Build history of the part. All positions in model axes, mm. A direction names the side the tool comes from. Round coordinates to 2 decimals unless told otherwise and drop trailing zeros. Order: outer loops, then holes, each group sorted by start corner. A loop starts at its lowest first (then second) coordinate and runs counter-clockwise, first axis right, second up. Notation, with made-up numbers: (22.25, 2.25) -> (59.25, 2.25) arc R30 ccw to (59.25, 33.25) -> close; hole circle Ø8 at (75, 81.25). An arc over 180 degrees is marked (long way). Answer as a JSON object with one key per item and string values.
from build123d import *

# Parameters (mm, degrees)
F0_W      = 85
F0_H      = 85
F0_R      = 2
F3_DEPTH  = 18.5
F4_DEPTH  = 14
F5_R      = 5
F6_R      = 3
F7_R      = 1
F8_R      = 3.1
F9_DEPTH  = 3.1
F10_R     = 3.1
F11_DEPTH = 3.1
F12_R     = 3.1
F13_DEPTH = 3.1
F14_R     = 3.1
F15_DEPTH = 3.1
F16_DEPTH = 1
F17_ANGLE = 180


# Not quite as in the source:
# - a feature names something its author has since deleted; it is built from what else it names


with BuildPart() as f3:
    # F0 (on Top) → F3 (new body)
    with BuildSketch(Plane.XY):
        Rectangle(F0_W, F0_H)
        with Locations((0, -37.75)):
            Circle(F0_R, mode=Mode.SUBTRACT)
        with BuildLine():
            ThreePointArc((-33, 30), (-32.1213203436, 32.1213203436), (-30, 33))
            Line((-30, 33), (30, 33))
            ThreePointArc((30, 33), (32.1213203436, 32.1213203436), (33, 30))
            Line((33, 30), (33, -30))
            ThreePointArc((33, -30), (32.1213203436, -32.1213203436), (30, -33))
            Line((30, -33), (-30, -33))
            ThreePointArc((-30, -33), (-32.1213203436, -32.1213203436), (-33, -30))
            Line((-33, -30), (-33, 30))
        make_face(mode=Mode.SUBTRACT)
        with BuildLine():
            Line((30, 33), (-30, 33))
            ThreePointArc((-30, 33), (-32.1213203436, 32.1213203436), (-33, 30))
            Line((-33, 30), (-33, -30))
            ThreePointArc((-33, -30), (-32.1213203436, -32.1213203436), (-30, -33))
            Line((-30, -33), (30, -33))
            ThreePointArc((30, -33), (32.1213203436, -32.1213203436), (33, -30))
            Line((33, -30), (33, 30))
            ThreePointArc((33, 30), (32.1213203436, 32.1213203436), (30, 33))
        make_face()
        with Locations((0, -37.75)):
            Circle(F0_R)
    extrude(amount=F3_DEPTH)

    # F0 (on Top) → F4 (cut)
    with BuildSketch(Plane.XY):
        with BuildLine():
            Line((30, 33), (-30, 33))
            ThreePointArc((-30, 33), (-32.1213203436, 32.1213203436), (-33, 30))
            Line((-33, 30), (-33, -30))
            ThreePointArc((-33, -30), (-32.1213203436, -32.1213203436), (-30, -33))
            Line((-30, -33), (30, -33))
            ThreePointArc((30, -33), (32.1213203436, -32.1213203436), (33, -30))
            Line((33, -30), (33, 30))
            ThreePointArc((33, 30), (32.1213203436, 32.1213203436), (30, 33))
        make_face()
    extrude(amount=F4_DEPTH, mode=Mode.SUBTRACT)

    # F5
    f5_edges = [f3.edges().sort_by_distance(p)[0] for p in [
        (0, 42.5, 18.5),
        (-42.5, 0, 18.5),
        (0, -42.5, 18.5),
        (42.5, 0, 18.5),
        (42.5, 42.5, 9.25),
        (-42.5, 42.5, 9.25),
        (-42.5, -42.5, 9.25),
        (42.5, -42.5, 9.25),
    ]]
    fillet(f5_edges, radius=F5_R)

    # F6
    f6_edges = [f3.edges().sort_by_distance(p)[0] for p in [
        (0, 33, 14),
        (-32.12132, 32.12132, 14),
        (-33, 0, 14),
        (-32.12132, -32.12132, 14),
        (0, -33, 14),
        (32.12132, -32.12132, 14),
        (33, 0, 14),
        (32.12132, 32.12132, 14),
    ]]
    fillet(f6_edges, radius=F6_R)

    # F7
    f7_edges = [f3.edges().sort_by_distance(p)[0] for p in [
        (0, 42.5, 0),
        (41.035534, 41.035534, 0),
        (-41.035534, 41.035534, 0),
        (42.5, 0, 0),
        (-42.5, 0, 0),
        (41.035534, -41.035534, 0),
        (-41.035534, -41.035534, 0),
        (0, -42.5, 0),
        (0, 33, 0),
        (-32.12132, 32.12132, 0),
        (-33, 0, 0),
        (-32.12132, -32.12132, 0),
        (0, -33, 0),
        (32.12132, -32.12132, 0),
        (33, 0, 0),
        (32.12132, 32.12132, 0),
    ]]
    fillet(f7_edges, radius=F7_R)

    # F8 (on face) → F9 (cut)
    with BuildSketch(Plane.XZ.offset(42.5)):
        with Locations((0, 7)):
            Circle(F8_R)
    extrude(amount=-F9_DEPTH, mode=Mode.SUBTRACT)

    # F10 (on face) → F11 (cut)
    with BuildSketch(Plane(origin=(0, 42.5, 0), x_dir=(-1, 0, 0), z_dir=(0, 1, 0))):
        with Locations((0, 7)):
            Circle(F10_R)
    extrude(amount=-F11_DEPTH, mode=Mode.SUBTRACT)

    # F12 (on face) → F13 (cut)
    with BuildSketch(Plane(origin=(-42.5, 0, 0), x_dir=(0, -1, 0), z_dir=(-1, 0, 0))):
        with Locations((0, 7)):
            Circle(F12_R)
    extrude(amount=-F13_DEPTH, mode=Mode.SUBTRACT)

    # F14 (on face) → F15 (cut)
    with BuildSketch(Plane.YZ.offset(42.5)):
        with Locations((0, 7)):
            Circle(F14_R)
    extrude(amount=-F15_DEPTH, mode=Mode.SUBTRACT)

    # F0 (on Top) → F16 (cut)
    with BuildSketch(Plane.XY):
        with Locations((0, -37.75)):
            Circle(F0_R)
    extrude(amount=F16_DEPTH, mode=Mode.SUBTRACT)


with BuildPart() as f3_1:
    # F17: moved
    add(f3.part.rotate(Axis((0, 0, 0), (0, 1, 0)), F17_ANGLE))


solid = f3_1.part
1) Pull direction X, two halves, no side cores. Call faces 1 (the face through (-33, 0, -6)), 2 (the face through (1, 1, -18.5)), 3 (the face through (-41, 41.07, -7.34)): pulls with the +X half, pulls with the -X half, needs draft (parallel to the pull), parting line crosses it, or undercut.
Checked values:
{"face 1": "undercut", "face 2": "needs draft", "face 3": "pulls with the -X half"}
2) Probe L1, parallel to Y at x = -24.5, z = -6.5; L2, parallel to Y at x = 0, z = -0.4. List the from-to ranges inside material, lowest first. Write a range as from..to.
Checked values:
{"L1": "y = -42.5..-33, 33..42.5", "L2": "y = -42.3..-39.75, -35.75..-33.2, 33.2..42.3"}
3) Cut at C-C, the plane x = 0. Give the cut face in (y, z), plus the area to 3 significant figures.
Checked values:
{"outline": "(-42.5, -13.5) arc R5 ccw to (-37.5, -18.5) -> (37.5, -18.5) arc R5 ccw to (42.5, -13.5) -> (42.5, -10.1) -> (39.4, -10.1) -> (39.4, -3.9) -> (42.5, -3.9) -> (42.5, -1) arc R1 ccw to (41.5, 0) -> (34, 0) arc R1 ccw to (33, -1) -> (33, -11) arc R3 cw to (30, -14) -> (-30, -14) arc R3 cw to (-33, -11) -> (-33, -1) arc R1 ccw to (-34, 0) -> (-35.75, 0) -> (-35.75, -1) -> (-39.75, -1) -> (-39.75, 0) -> (-41.5, 0) arc R1 ccw to (-42.5, -1) -> (-42.5, -3.9) -> (-39.4, -3.9) -> (-39.4, -10.1) -> (-42.5, -10.1) -> close", "area": "598 mm²"}
4) Cut at D-D, the plane y = -23.5. Give the cut face in (x, z).
Checked values:
{"outline": "(-42.5, -13.5) arc R5 ccw to (-37.5, -18.5) -> (37.5, -18.5) arc R5 ccw to (42.5, -13.5) -> (42.5, -1) arc R1 ccw to (41.5, 0) -> (34, 0) arc R1 ccw to (33, -1) -> (33, -11) arc R3 cw to (30, -14) -> (-30, -14) arc R3 cw to (-33, -11) -> (-33, -1) arc R1 ccw to (-34, 0) -> (-41.5, 0) arc R1 ccw to (-42.5, -1) -> close"}
5) Which spindle directions (+Z, -Z, +X, -X, +Y, -Y) get a long thin tool onto all of the face, cutting with end or side? Do faces 4 (the face through (0, 39.4, -7)), 5 (the face through (32.1, 32.14, -5.93)), 6 (the face through (40.972, 0.404, -10.074)), 7 (the face through (2.46, -40.972, -5.114)). Say none if no direction does.
Checked values:
{"face 4": "+Y", "face 5": "+Z", "face 6": "+X", "face 7": "-Y"}
6) Cut at B-B, the plane y = 0. Give the cut face in (x, z).
Checked values:
{"outline": "(-42.5, -13.5) arc R5 ccw to (-37.5, -18.5) -> (37.5, -18.5) arc R5 ccw to (42.5, -13.5) -> (42.5, -10.1) -> (39.4, -10.1) -> (39.4, -3.9) -> (42.5, -3.9) -> (42.5, -1) arc R1 ccw to (41.5, 0) -> (34, 0) arc R1 ccw to (33, -1) -> (33, -11) arc R3 cw to (30, -14) -> (-30, -14) arc R3 cw to (-33, -11) -> (-33, -1) arc R1 ccw to (-34, 0) -> (-41.5, 0) arc R1 ccw to (-42.5, -1) -> (-42.5, -3.9) -> (-39.4, -3.9) -> (-39.4, -10.1) -> (-42.5, -10.1) -> close"}
7) Flat gauge pins, fed straight in: pin 1 Ø1.9 at (y, z) = (-1, -7) entering from -X; pin 2 Ø5.5 at (x, z) = (0, -7) entering from -Y; pin 3 Ø1 at (x, y) = (-16, -27.5) entering from +Z. Where does each tip first touch, or does it go through?
Checked values:
{"pin 1": "stops at x = -39.4", "pin 2": "stops at y = -39.4", "pin 3": "stops at z = -14"}
